from build123d import *

# Parameters (mm, degrees)
SKETCH_1_W      = 22.5
SKETCH_1_H      = 20
SKETCH_1_R      = 1.5
EXTRUDE_1_DEPTH = 1.5
SKETCH_1_3_R    = 5.85
EXTRUDE_2_DEPTH = 8.84
SKETCH_1_4_W    = 2.5
SKETCH_1_4_H    = 8
EXTRUDE_3_DEPTH = 4


with BuildPart() as part:
    # Sketch 1 → Extrude 1 (new body)
    with BuildSketch(Plane(origin=(0, 0, 0), x_dir=(1, 0, 0), z_dir=(0, 1, 0))):
        with Locations((11.25, 10)):
            Rectangle(SKETCH_1_W, SKETCH_1_H)
        with Locations(Location((2, 18, 0), (0, 0, 270))):
            Circle(SKETCH_1_R, mode=Mode.SUBTRACT)
        with Locations(Location((2, 2, 0), (0, 0, 270))):
            Circle(SKETCH_1_R, mode=Mode.SUBTRACT)
        with Locations(Location((20.5, 2, 0), (0, 0, 270))):
            Circle(SKETCH_1_R, mode=Mode.SUBTRACT)
        with Locations(Location((20.5, 18, 0), (0, 0, 270))):
            Circle(SKETCH_1_R, mode=Mode.SUBTRACT)
    extrude(amount=-EXTRUDE_1_DEPTH)

    # Sketch 1_3 → Extrude 2 (add)
    with BuildSketch(Plane(origin=(0, 0, 0), x_dir=(1, 0, 0), z_dir=(0, 1, 0))):
        with Locations(Location((13, 10, 0), (0, 0, 270))):
            Circle(SKETCH_1_3_R)
    extrude(amount=EXTRUDE_2_DEPTH)

    # Sketch 1_4 → Extrude 3 (add)
    with BuildSketch(Plane(origin=(0, 0, 0), x_dir=(1, 0, 0), z_dir=(0, 1, 0))):
        with Locations((1.25, 10)):
            Rectangle(SKETCH_1_4_W, SKETCH_1_4_H)
    extrude(amount=EXTRUDE_3_DEPTH)


solid = part.part
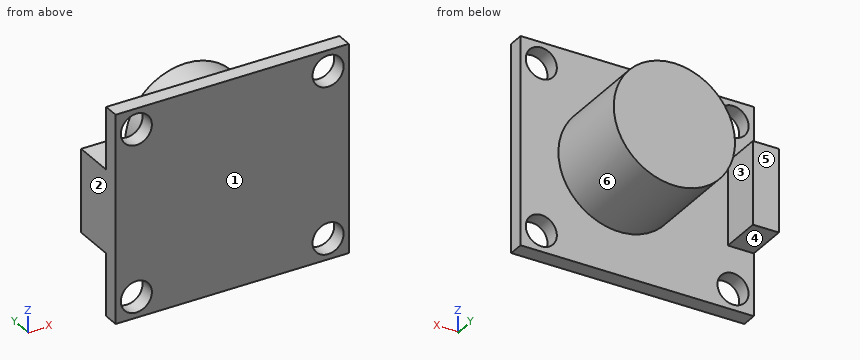
Work out the finished part from the listing and answer in its coordinate system (mm). Face numbers are marked on the shaded views. A direction names the side the tool comes from. Coordinates: 2 decimals unless noted, no trailing zeros. Write each loop counter-clockwise with the first axis right and the second up, starting at its lowest first coordinate (ties: lowest second). Pieces come first, ordered by that corner, then holes. Notation, with made-up numbers: M 35,38 L 45,38 A11 ccw 45,47 Z; hole C -37.75,36 d8. An arc over 180 degrees is marked long. Use one line per item in the form item = value. Start each with the question number.
1. A tool of negligible diameter and unlimited length cuts with its end or side. For the marked faces 4, 5 and 6, from which of +Z, -Z, +X, -X, +Y, -Y can it reach the whole face along a straight path? Write none if from no direction.
2. Straight lines are drawn through the part: probe 1 along X at (y, z) = (-0.4, -2); probe 2 along Z at (x, y) = (2, 1.5); probe 3 along Y at (x, z) = (2, -10.5). For each, find the intervals that lie inside material, in ascending order. Write a range as from..to.
3. Each of these flat-tipped pins is pushed along its axis until it touches: P1, Ø0.8, axis at x = 1, z = -9, coming from the +Y side; P2, Ø2, axis at y = 6, z = -7, coming from the +X side; P3, Ø3, axis at x = 1.5, y = 2, coming from the -Z side; P4, Ø2, axis at x = 14.5, y = 0.5, coming from the -Z side. Where does it stop, or does it pass through?
4. The part is cut by section D-D (x = 13). Give the vertices of the cut face in (y, z), plus the area to 3 significant figures.
5. The part is cut by section B-B (x = 20.5). Give the vertices of the cut face in (y, z).
6. The part is cut by section C-C (y = 2). Give the vertices of the cut face in (x, z), plus the area to 3 significant figures.
7. The mould has two halves that part along X. Classify the marked faces 1, 2 and 3: released by +X, released by -X, zero draft, split by the parting line, or undercut.
8. The part is cut by section A-A (z = -18). Give the vertices of the cut face in (x, y), plus the area to 4 significant figures.
Evaluation:
q1.face_4 = -Z, -X, +Y
q1.face_5 = +Z, -Z, -X, +Y
q1.face_6 = +Y
q2.probe_1 = 0..0.5, 3.5..19, 22..22.5
q2.probe_2 = -14..-6
q2.probe_3 = -1.5..4
q3.P1 = 4
q3.P2 = 18.5
q3.P3 = -14
q3.P4 = -20
q4.outline = M -1.5,-20 L 0,-20 L 0,-15.85 L 8.84,-15.85 L 8.84,-4.15 L 0,-4.15 L 0,0 L -1.5,0 Z
q4.area = 133 mm^2
q5.outline = M -1.5,-20 L 0,-20 L 0,-19.5 L -1.5,-19.5 Z; M -1.5,-16.5 L 0,-16.5 L 0,-3.5 L -1.5,-3.5 Z; M -1.5,-0.5 L 0,-0.5 L 0,0 L -1.5,0 Z
q6.outline = M 0,-14 L 2.5,-14 L 2.5,-6 L 0,-6 Z; C 13,-10 d11.7
q6.area = 128 mm^2
q7.face_1 = zero draft
q7.face_2 = released by -X
q7.face_3 = undercut
q8.outline = M 0,-1.5 L 0.5,-1.5 L 0.5,0 L 0,0 Z; M 3.5,-1.5 L 19,-1.5 L 19,0 L 3.5,0 Z; M 22,-1.5 L 22.5,-1.5 L 22.5,0 L 22,0 Z
q8.area = 24.75 mm^2
